The model under review builds one solid part; all positions refer to its coordinate system, in mm. Round coordinates to 2 decimals unless told otherwise and drop trailing zeros. Loops run counter-clockwise (first coordinate to the right, second up) from the corner with the lowest first, then second, coordinate; pieces in that order, holes last. Notation, with made-up numbers: M 66,-29.5 L 98,-29.5 A12 ccw 98,-8.5 Z; hole C 86,38.5 d1. An arc over 180 degrees is marked long. Return JSON: item names as keys, results as strings. Group by question number.
Q1. Consider section A-A (y = 32). State the section outline as (x, z) points (3 decimals), and give its area (4 significant figures).
Q2. Clearance check with flat-ended pins moving along their axes: pin 1 Ø1 at (x, y) = (1.5, 21) entering from +Z; pin 2 Ø1 at (x, z) = (0.5, 34.5) entering from -Y. State where each tip first meets the part, or that it passes through.
Q3. To check wall thickness, follow line 1 along Y through (x, z) = (2.2, -2.5); line 2 along Z through (x, y) = (2.4, -31) (3 decimals); line 3 along Y through (x, z) = (0.95, -40.5). State the ranges of each line that lie inside material, in increasing order.
Q4. Consider section B-B (z = -35). State the section outline as (x, y) points (1 decimal).
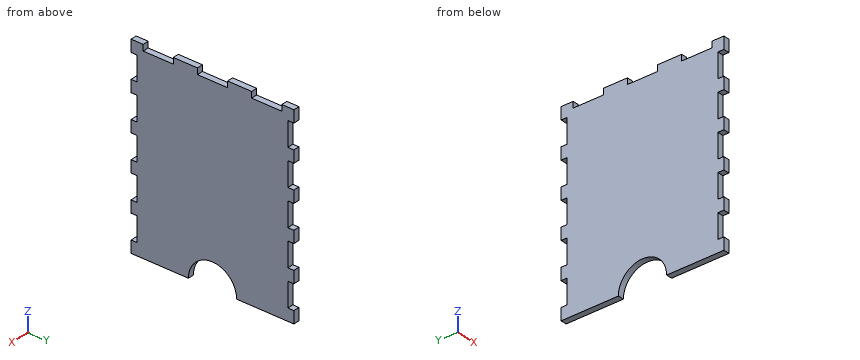
from build123d import *

# Parameters (mm, degrees)
F0_W     = 85.725
F0_H     = 101.6
F1_DEPTH = 3.175
F2_W     = 3.175
F2_H     = 12.7
F3_DEPTH = 3.176
F4_W     = 15.875
F4_H     = 3.175
F5_DEPTH = 3.176
F7_DEPTH = 3.176


with BuildPart() as f1:
    # F0 (on Right) → F1 (new body)
    with BuildSketch(Plane.YZ):
        Rectangle(F0_W, F0_H)
    extrude(amount=F1_DEPTH)

    # F2 (on face) → F3 (cut, through all)
    with BuildSketch(Plane.YZ.offset(3.175)):
        with Locations((-41.275, -38.1)):
            Rectangle(F2_W, F2_H)
        with Locations((-41.275, -19.05)):
            Rectangle(F2_W, F2_H)
        with Locations((-41.275, 0)):
            Rectangle(F2_W, F2_H)
        with Locations((-41.275, 19.05)):
            Rectangle(F2_W, F2_H)
        with Locations((-41.275, 38.1)):
            Rectangle(F2_W, F2_H)
        with Locations((41.275, -38.1)):
            Rectangle(F2_W, F2_H)
        with Locations((41.275, -19.05)):
            Rectangle(F2_W, F2_H)
        with Locations((41.275, 38.1)):
            Rectangle(F2_W, F2_H)
        with Locations((41.275, 19.05)):
            Rectangle(F2_W, F2_H)
        with Locations((41.275, 0)):
            Rectangle(F2_W, F2_H)
    extrude(amount=-F3_DEPTH, mode=Mode.SUBTRACT)

    # F4 (on face) → F5 (cut, through all)
    with BuildSketch(Plane.YZ.offset(3.175)):
        with Locations((-28.575, 49.2125)):
            Rectangle(F4_W, F4_H)
        with Locations((0, 49.2125)):
            Rectangle(F4_W, F4_H)
        with Locations((28.575, 49.2125)):
            Rectangle(F4_W, F4_H)
    extrude(amount=-F5_DEPTH, mode=Mode.SUBTRACT)

    # F6 (on face) → F7 (cut, through all)
    with BuildSketch(Plane.YZ.offset(3.175)):
        with BuildLine():
            add(Edge.make_bspline(
                [(12.7, -50.8), (12.7, -28.802955), (-6.35, -39.801477), (-25.4, -50.8), (-6.35, -61.798523), (12.7, -72.797045), (12.7, -50.8)],
                knots=[0, 0, 0, 2.094395, 2.094395, 4.18879, 4.18879, 6.283185, 6.283185, 6.283185], degree=2, weights=[1, 0.5, 1, 0.5, 1, 0.5, 1]))
        make_face()
    extrude(amount=-F7_DEPTH, mode=Mode.SUBTRACT)


solid = f1.part
Values:
{
 "1": {"outline": "M 0,-50.8 L 3.175,-50.8 L 3.175,47.625 L 0,47.625 Z", "area": "312.5 mm2"},
 "2": {"pin 1": "stops at z = 50.8", "pin 2": "stops at y = -39.69"},
 "3": {"line 1": "y = -39.69 to 39.69", "line 2": "z = -50.8 to 47.625", "line 3": "y = -39.69 to -7.43, 7.43 to 39.69"},
 "4": {"outline": "M 0,-39.7 L 3.2,-39.7 L 3.2,39.7 L 0,39.7 Z"}
}
